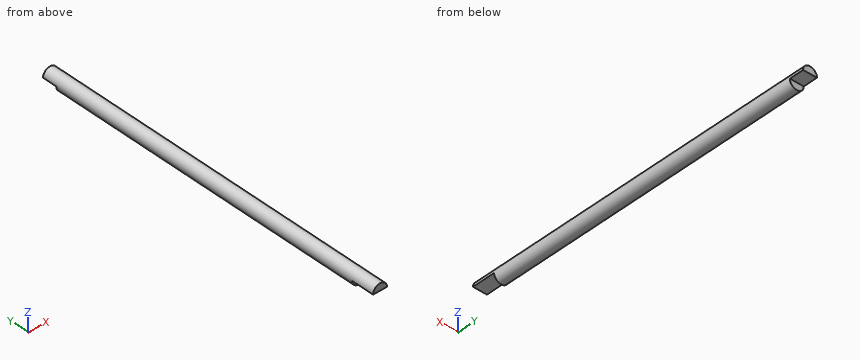
```python
from build123d import *

# Parameters (mm, degrees)
SKETCH1_R           = 1.95
BOSS_EXTRUDE1_DEPTH = 50
SKETCH2_W           = 3.9
SKETCH2_H           = 4
SKETCH2_H_2         = 6.4
CUT_EXTRUDE1_DEPTH  = 51.075992252


with BuildPart() as part:
    # Sketch1 → Boss-Extrude1 (new, symmetric)
    with BuildSketch(Plane(origin=(0, 0, 0), x_dir=(1, 0, 0), z_dir=(0, 1, 0))):
        with Locations(Location((0, 0, 0), (0, 0, 270))):
            Circle(SKETCH1_R)
    extrude(amount=BOSS_EXTRUDE1_DEPTH, both=True)

    # Sketch2 → Cut-Extrude1 (cut, through all)
    with BuildSketch(Plane.XY):
        with Locations((0, 48)):
            Rectangle(SKETCH2_W, SKETCH2_H)
        with Locations((0, -46.8)):
            Rectangle(SKETCH2_W, SKETCH2_H_2)
    extrude(amount=-CUT_EXTRUDE1_DEPTH, mode=Mode.SUBTRACT)


solid = part.part
```
Build history of the part. All positions in model axes, mm. Give positions to 0.01 mm unless a question says otherwise; leave off trailing zeros. Loops run counter-clockwise (first coordinate to the right, second up) from the corner with the lowest first, then second, coordinate; pieces in that order, holes last. Notation, with made-up numbers: (26.5, 77.5) - (39.5, 77.5) arc R15 cw to (39.5, 103.5) - close; hole circle Ø5 at (-4, -29). An arc over 180 degrees is marked (long way). Use a Markdown table: item, result.
(1) Band-saw the part on C-C (z = -1.25). Give the cut face in (x, y).
Taken from the geometry:
| item | result |
|---|---|
| outline | (-1.5, -43.6) - (1.5, -43.6) - (1.5, 46) - (-1.5, 46) - close |
(2) Drop flat-ended pins along their axis: pin 1 Ø1.5 at (y, z) = (-14, -0.5) entering from -X; pin 2 Ø1 at (x, z) = (0, -1) entering from -Y; pin 3 Ø1.2 at (x, y) = (0.5, 48.5) entering from -Z. Give the stop position or say it passes through.
Taken from the geometry:
| item | result |
|---|---|
| pin 1 | x = -1.95 |
| pin 2 | y = -43.6 |
| pin 3 | z = 0 |
(3) Band-saw the part on B-B (y = -24). Give the cut face in (x, z).
Taken from the geometry:
| item | result |
|---|---|
| outline | circle Ø3.9 at (0, 0) |
(4) Wall check: line 1 along Y through (x, z) = (-0.2, -1.1); line 2 along Z through (x, y) = (0.1, -44); line 3 along X through (y, z) = (44.5, -0.1). Give the ranges that are in metal, low to high.
Taken from the geometry:
| item | result |
|---|---|
| line 1 | -43.6 to 46 |
| line 2 | 0 to 1.95 |
| line 3 | -1.95 to 1.95 |
(5) Band-saw the part on A-A (x = 0). Give the cut face in (y, z), and give its area (3 significant figures).
Taken from the geometry:
| item | result |
|---|---|
| outline | (-50, 0) - (-43.6, 0) - (-43.6, -1.95) - (46, -1.95) - (46, 0) - (50, 0) - (50, 1.95) - (-50, 1.95) - close |
| area | 370 mm2 |
